from build123d import *

# Parameters (mm, degrees)
SKETCH2_R           = 2.6035
BOSS_EXTRUDE1_DEPTH = 3.175
FILLET1_R           = 7.62


with BuildPart() as part:
    # Sketch2 → Boss-Extrude1 (new body)
    with BuildSketch(Plane.XY):
        Polygon((0, -9.525), (0, 9.525), (-108.669578778, 9.525), (-165.682370629, 57.364412615), (-177.927474593, 42.771265973), (-115.60321174, -9.525), align=None)
        with Locations((-164.021911069, 43.53711718)):
            Circle(SKETCH2_R, mode=Mode.SUBTRACT)
        with Locations((-115.378088931, 2.720103965)):
            Circle(SKETCH2_R, mode=Mode.SUBTRACT)
        with Locations((-73.66, 0)):
            Circle(SKETCH2_R, mode=Mode.SUBTRACT)
        with Locations((-44.45, 0)):
            Circle(SKETCH2_R, mode=Mode.SUBTRACT)
        with Locations((-15.24, 0)):
            Circle(SKETCH2_R, mode=Mode.SUBTRACT)
    extrude(amount=BOSS_EXTRUDE1_DEPTH)

    # Fillet1
    fillet1_edges = [part.edges().sort_by_distance(p)[0] for p in [
        (-115.60321174, -9.525, 1.5875),
        (-177.927474593, 42.771265973, 1.5875),
        (-165.682370629, 57.364412615, 1.5875),
        (-108.669578778, 9.525, 1.5875),
        (0, 9.525, 1.5875),
        (0, -9.525, 1.5875),
    ]]
    fillet(fillet1_edges, radius=FILLET1_R)


solid = part.part
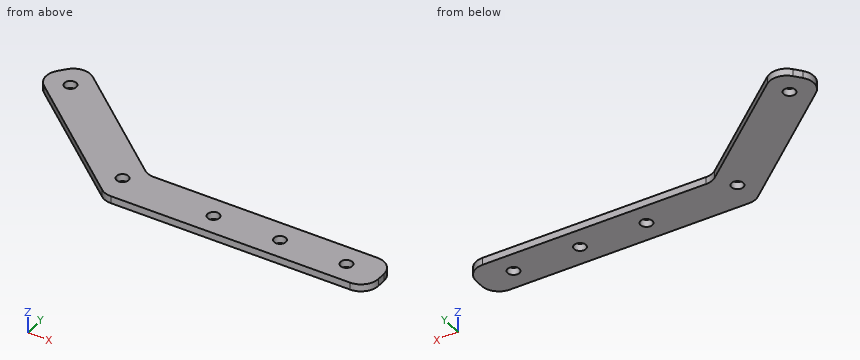
Part model, mm, in its own coordinate system. Coordinates: 2 decimals unless noted, no trailing zeros. Write each loop counter-clockwise with the first axis right and the second up, starting at its lowest first coordinate (ties: lowest second). Pieces come first, ordered by that corner, then holes. Notation, with made-up numbers: (7, -39.75) - (18, -39.75) arc R16 cw to (18, -23.75) - close; hole circle Ø10 at (-37.75, 85.25). An arc over 180 degrees is marked (long way). Put each result on its own line as item: value.
1. Flat gauge pins, fed straight in: pin 1 Ø1 at (x, z) = (-114.5, 2) entering from +Y; pin 2 Ø1.6 at (x, z) = (-72, 2) entering from +Y (3 decimals); pin 3 Ø1 at (y, z) = (39.5, 2.5) entering from +X. Where does each tip first touch, or does it go through?
Final values:
pin 1: stops at y = 14.84
pin 2: stops at y = 9.525
pin 3: stops at x = -143.8
2. Probe line 1 along Y through (x, z) = (-44.45, 0.8) (1 decimal); line 2 along Y through (x, z) = (-38, 2.15) (3 decimals); line 3 along X through (y, z) = (-2, 2.55). List the from-to ranges inside material, lowest first. Write a range as [from, to].
Final values:
line 1: y = [-9.5, -2.6], [2.6, 9.5]
line 2: y = [-9.525, 9.525]
line 3: x = [-124.57, -75.33], [-71.99, -46.12], [-42.78, -16.91], [-13.57, 0]
3. Band-saw the part on D-D (x = -128). Write the cut outline in (y, z) (3 decimals), then the cut area to 3 significant figures.
Final values:
outline: (0.877, 0) - (25.745, 0) - (25.745, 3.175) - (0.877, 3.175) - close
area: 79.0 mm²
4. Band-saw the part on C-C (y = 35). Write the cut outline in (x, z) (1 decimal).
Final values:
outline: (-168.7, 0) - (-139, 0) - (-139, 3.2) - (-168.7, 3.2) - close
5. Band-saw the part on B-B (z = 0.9). Give the number of separate pieces and of enclosed holes in the cut face, then the cut area to 3 significant figures.
Final values:
separate pieces: 1
enclosed holes: 5
area: 3,460 mm²
6. Band-saw the part on A-A (x = -73.66). Write the cut outline in (y, z) (1 decimal).
Final values:
outline: (-9.5, 0) - (-2.6, 0) - (-2.6, 3.2) - (-9.5, 3.2) - close; (2.6, 0) - (9.5, 0) - (9.5, 3.2) - (2.6, 3.2) - close
